from build123d import *

# Parameters (mm, degrees)
SKETCH1_W           = 25
SKETCH1_H           = 20
BOSS_EXTRUDE1_DEPTH = 12
SKETCH2_R           = 2.25
CUT_EXTRUDE1_DEPTH  = 64.237868143


with BuildPart() as part:
    # Sketch1 → Boss-Extrude1 (new body)
    with BuildSketch(Plane(origin=(0, 0, 0), x_dir=(1, 0, 0), z_dir=(0, 1, 0))):
        Polygon((-47.833335, 15), (47.833335, 15), (47.833335, 10), (56.833335, 10), (56.833335, -10), (47.833335, -10), (47.833335, -15), (-47.833335, -15), (-47.833335, -10), (-56.833335, -10), (-56.833335, 10), (-47.833335, 10), align=None)
        with Locations((-21.115289313, 0)):
            Rectangle(SKETCH1_W, SKETCH1_H, mode=Mode.SUBTRACT)
        with Locations((21.115289313, 0)):
            Rectangle(SKETCH1_W, SKETCH1_H, mode=Mode.SUBTRACT)
    extrude(amount=BOSS_EXTRUDE1_DEPTH)

    # Sketch2 → Cut-Extrude1 (cut, through all)
    with BuildSketch(Plane(origin=(0, 0, -10), x_dir=(-1, 0, 0), z_dir=(0, 0, -1))):
        with Locations((-51.833335, 6)):
            Circle(SKETCH2_R)
        with Locations((51.833335, 6)):
            Circle(SKETCH2_R)
    extrude(amount=-CUT_EXTRUDE1_DEPTH, mode=Mode.SUBTRACT)


solid = part.part
Geometry: final body of the model. Coordinates: model frame, mm. A direction names the side the tool comes from. Coordinates: 2 decimals unless noted, no trailing zeros. Loops run counter-clockwise (first coordinate to the right, second up) from the corner with the lowest first, then second, coordinate; pieces in that order, holes last. Notation, with made-up numbers: M 49,-21 L 62,-21 A19 cw 62,-9 Z; hole C -8.75,65 d1. An arc over 180 degrees is marked long. One line per item, written item: value. Start each with the question number.
1) Cut plane D-D (y = 1.75). Return loops of the section in (x, z).
2) Cut plane B-B (z = 4). Return loops of the section in (x, y), then the cut area to 3 significant figures.
3) Draft query along X for faces 1 (the flat face through (21, 6, -10)), 2 (the flat face through (-54.4, 5.9, -10)), 3 (the flat face through (56.833, 6, 0)), 4 (the flat face through (21, 6, 10)). Return one class per face: released by +X, released by -X, zero draft, split by the parting line, or undercut.
4) Pin query (flat end, axial travel): P1, Ø5.5, axis at y = 7, z = 12, coming from the -X side; P2, Ø4, axis at y = 5, z = 13, coming from the +X side; P3, Ø7, axis at x = 54, y = 4.5, coming from the +Z side; P4, Ø5.5, axis at y = 8.5, z = -13, coming from the -X side. Return the tip coordinate at first contact, or that it passes through.
5) Material intervals for L1, parallel to X at y = 8.5, z = -8.75; L2, parallel to Z at x = 11.5, y = 9.75; L3, parallel to X at y = 6.75, z = -8.5, sorted ascending. Write a range as from..to.
6) Cut plane C-C (x = -20.5). Return loops of the section in (y, z), then the cut area to 3 significant figures.
7) Reachability of faces 5 (the flat face through (8.615, 6, 0)), 6 (the flat face through (47.833, 6, 12)), 7 (the flat face through (-47.833, 6, -12)), 8 (the flat face through (54.3, 5.9, -10)), 9 (the flat face through (-54.3, 5.9, 10)) from +Z, -Z, +X, -X, +Y, -Y: full face, straight path, thin tool, end or side. Return the list, or none.
8) Cut plane A-A (y = 6). Return loops of the section in (x, z).
Evaluation:
1. outline: M -56.83,-10 L -47.83,-10 L -47.83,-15 L 47.83,-15 L 47.83,-10 L 56.83,-10 L 56.83,10 L 47.83,10 L 47.83,15 L -47.83,15 L -47.83,10 L -56.83,10 Z; hole M -33.62,-10 L -8.62,-10 L -8.62,10 L -33.62,10 Z; hole M 8.62,-10 L 33.62,-10 L 33.62,10 L 8.62,10 Z
2. outline: M -56.83,0 L -33.62,0 L -33.62,12 L -56.83,12 Z; M -8.62,0 L 8.62,0 L 8.62,12 L -8.62,12 Z; M 33.62,0 L 56.83,0 L 56.83,12 L 33.62,12 Z; hole C -51.83,6 d4.5; hole C 51.83,6 d4.5
2. area: 732 mm^2
3. face 1: undercut
3. face 2: zero draft
3. face 3: released by +X
3. face 4: undercut
4. P1: x = -56.83
4. P2: x = 47.83
4. P3: z = 10
4. P4: x = -47.83
5. L1: -56.83..-33.62, -8.62..8.62, 33.62..56.83
5. L2: -15..-10, 10..15
5. L3: -56.83..-53.95, -49.71..-33.62, -8.62..8.62, 33.62..49.71, 53.95..56.83
6. outline: M 0,-15 L 12,-15 L 12,-10 L 0,-10 Z; M 0,10 L 12,10 L 12,15 L 0,15 Z
6. area: 120 mm^2
7. face 5: +Y, -Y
7. face 6: +Z, +X, +Y, -Y
7. face 7: -Z, -X, +Y, -Y
7. face 8: -Z, +X, +Y, -Y
7. face 9: +Z, -X, +Y, -Y
8. outline: M -56.83,-10 L -54.08,-10 L -54.08,10 L -56.83,10 Z; M -49.58,-10 L -47.83,-10 L -47.83,-15 L 47.83,-15 L 47.83,-10 L 49.58,-10 L 49.58,10 L 47.83,10 L 47.83,15 L -47.83,15 L -47.83,10 L -49.58,10 Z; M 54.08,-10 L 56.83,-10 L 56.83,10 L 54.08,10 Z; hole M -33.62,-10 L -8.62,-10 L -8.62,10 L -33.62,10 Z; hole M 8.62,-10 L 33.62,-10 L 33.62,10 L 8.62,10 Z
